Source: CAD feature listing. Evaluate the final solid. Frame: model axes, mm. Face numbers are marked on the shaded views. A direction names the side the tool comes from. Coordinates: 2 decimals unless noted, no trailing zeros. Order: outer loops, then holes, each group sorted by start corner. A loop starts at its lowest first (then second) coordinate and runs counter-clockwise, first axis right, second up.
Item 1: Mould query, pull axis X, two halves, no side actions, for the marked faces 4, 5 and 6. Classes: released by +X, released by -X, zero draft, split by the parting line, or undercut.
Item 2: Section B-B on z = 17. Return the cut outline in (x, y), then the cut area to 3 significant figures.
Item 3: Section A-A on y = 14.05. Return the cut outline in (x, z) (3 decimals), then the cut area to 3 significant figures.
Item 4: Ray query, line 1 (Z direction, x = 7.5, y = 13.6) (3 decimals); line 2 (Z direction, x = 5.5, y = 14.1); line 3 (Z direction, x = 6.75, y = 16.95). Return the intervals inside material, ascending.
Item 5: Section D-D on z = 13.25. Return the cut outline in (x, y).
Item 6: Section C-C on y = 15.3. Return the cut outline in (x, z) (3 decimals).
Item 7: Reachability of the marked faces 1, 2 and 3 from +Z, -Z, +X, -X, +Y, -Y: full face, straight path, thin tool, end or side. Return the list, or none.
Item 8: Contact query for flat-ended pins moving along their axis: P1, Ø8, axis at x = 12.5, z = -4.5, coming from the +Y side; P2, Ø4, axis at x = 8.6, z = 14.5, coming from the -Y side; P3, Ø0.9, axis at x = 12.5, y = 17, coming from the +Z side. Output: stop coordinate, or through.
from build123d import *

# Parameters (mm, degrees)
BOSS_EXTRUDE1_DEPTH  = 9
SKETCH6_W            = 16
SKETCH6_H            = 9
BOSS_EXTRUDE6_DEPTH  = 2.75
SKETCH7_W            = 16
SKETCH7_H            = 2.75
BOSS_EXTRUDE7_DEPTH  = 10
SKETCH8_W            = 16
SKETCH8_H            = 2.75
BOSS_EXTRUDE8_DEPTH  = 10
SKETCH10_R           = 1.625
CUT_EXTRUDE1_DEPTH   = 10
CUT_EXTRUDE2_DEPTH   = 1.5
BOSS_EXTRUDE11_DEPTH = 0.3


with BuildPart() as part:
    # Sketch1 → Boss-Extrude1 (new body)
    with BuildSketch(Plane.XY):
        with BuildLine():
            Line((16.338025278, 17.821295042), (16.597849853, 17.821295042))
            Line((16.597849853, 17.821295042), (16.597849853, 15.951295042))
            Line((16.597849853, 15.951295042), (0.597849853, 15.951295042))
            Line((0.597849853, 15.951295042), (0.597849853, 17.821295042))
            Line((0.597849853, 17.821295042), (0.857674428, 17.821295042))
            ThreePointArc((0.857674428, 17.821295042), (0.956581499, 17.784066453), (1.006392961, 17.690860259))
            ThreePointArc((1.006392961, 17.690860259), (1.040238138, 17.533232888), (1.098973448, 17.383092794))
            ThreePointArc((1.098973448, 17.383092794), (1.303700441, 17.155655983), (1.597849853, 17.071295042))
            ThreePointArc((1.597849853, 17.071295042), (1.891999264, 17.155655983), (2.096726257, 17.383092794))
            ThreePointArc((2.096726257, 17.383092794), (2.155461567, 17.533232888), (2.189306744, 17.690860259))
            ThreePointArc((2.189306744, 17.690860259), (2.239118207, 17.784066453), (2.338025278, 17.821295042))
            Line((2.338025278, 17.821295042), (2.857674428, 17.821295042))
            ThreePointArc((2.857674428, 17.821295042), (2.956581499, 17.784066453), (3.006392961, 17.690860259))
            ThreePointArc((3.006392961, 17.690860259), (3.040238138, 17.533232888), (3.098973448, 17.383092794))
            ThreePointArc((3.098973448, 17.383092794), (3.303700441, 17.155655983), (3.597849853, 17.071295042))
            ThreePointArc((3.597849853, 17.071295042), (3.891999264, 17.155655983), (4.096726257, 17.383092794))
            ThreePointArc((4.096726257, 17.383092794), (4.155461567, 17.533232888), (4.189306744, 17.690860259))
            ThreePointArc((4.189306744, 17.690860259), (4.239118207, 17.784066453), (4.338025278, 17.821295042))
            Line((4.338025278, 17.821295042), (4.857674428, 17.821295042))
            ThreePointArc((4.857674428, 17.821295042), (4.956581499, 17.784066453), (5.006392961, 17.690860259))
            ThreePointArc((5.006392961, 17.690860259), (5.040238138, 17.533232888), (5.098973448, 17.383092794))
            ThreePointArc((5.098973448, 17.383092794), (5.303700441, 17.155655983), (5.597849853, 17.071295042))
            ThreePointArc((5.597849853, 17.071295042), (5.891999264, 17.155655983), (6.096726257, 17.383092794))
            ThreePointArc((6.096726257, 17.383092794), (6.155461567, 17.533232888), (6.189306744, 17.690860259))
            ThreePointArc((6.189306744, 17.690860259), (6.239118207, 17.784066453), (6.338025278, 17.821295042))
            Line((6.338025278, 17.821295042), (6.857674428, 17.821295042))
            ThreePointArc((6.857674428, 17.821295042), (6.956581499, 17.784066453), (7.006392961, 17.690860259))
            ThreePointArc((7.006392961, 17.690860259), (7.040238138, 17.533232888), (7.098973448, 17.383092794))
            ThreePointArc((7.098973448, 17.383092794), (7.303700441, 17.155655983), (7.597849853, 17.071295042))
            ThreePointArc((7.597849853, 17.071295042), (7.891999264, 17.155655983), (8.096726257, 17.383092794))
            ThreePointArc((8.096726257, 17.383092794), (8.155461567, 17.533232888), (8.189306744, 17.690860259))
            ThreePointArc((8.189306744, 17.690860259), (8.239118207, 17.784066453), (8.338025278, 17.821295042))
            Line((8.338025278, 17.821295042), (8.857674428, 17.821295042))
            ThreePointArc((8.857674428, 17.821295042), (8.956581499, 17.784066453), (9.006392961, 17.690860259))
            ThreePointArc((9.006392961, 17.690860259), (9.040238138, 17.533232888), (9.098973448, 17.383092794))
            ThreePointArc((9.098973448, 17.383092794), (9.303700441, 17.155655983), (9.597849853, 17.071295042))
            ThreePointArc((9.597849853, 17.071295042), (9.891999264, 17.155655983), (10.096726257, 17.383092794))
            ThreePointArc((10.096726257, 17.383092794), (10.155461567, 17.533232888), (10.189306744, 17.690860259))
            ThreePointArc((10.189306744, 17.690860259), (10.239118207, 17.784066453), (10.338025278, 17.821295042))
            Line((10.338025278, 17.821295042), (10.857674428, 17.821295042))
            ThreePointArc((10.857674428, 17.821295042), (10.956581499, 17.784066453), (11.006392961, 17.690860259))
            ThreePointArc((11.006392961, 17.690860259), (11.040238138, 17.533232888), (11.098973448, 17.383092794))
            ThreePointArc((11.098973448, 17.383092794), (11.303700441, 17.155655983), (11.597849853, 17.071295042))
            ThreePointArc((11.597849853, 17.071295042), (11.891999264, 17.155655983), (12.096726257, 17.383092794))
            ThreePointArc((12.096726257, 17.383092794), (12.155461567, 17.533232888), (12.189306744, 17.690860259))
            ThreePointArc((12.189306744, 17.690860259), (12.239118207, 17.784066453), (12.338025278, 17.821295042))
            Line((12.338025278, 17.821295042), (12.857674428, 17.821295042))
            ThreePointArc((12.857674428, 17.821295042), (12.956581499, 17.784066453), (13.006392961, 17.690860259))
            ThreePointArc((13.006392961, 17.690860259), (13.040238138, 17.533232888), (13.098973448, 17.383092794))
            ThreePointArc((13.098973448, 17.383092794), (13.303700441, 17.155655983), (13.597849853, 17.071295042))
            ThreePointArc((13.597849853, 17.071295042), (13.891999264, 17.155655983), (14.096726257, 17.383092794))
            ThreePointArc((14.096726257, 17.383092794), (14.155461567, 17.533232888), (14.189306744, 17.690860259))
            ThreePointArc((14.189306744, 17.690860259), (14.239118207, 17.784066453), (14.338025278, 17.821295042))
            Line((14.338025278, 17.821295042), (14.857674428, 17.821295042))
            ThreePointArc((14.857674428, 17.821295042), (14.956581499, 17.784066453), (15.006392961, 17.690860259))
            ThreePointArc((15.006392961, 17.690860259), (15.040238138, 17.533232888), (15.098973448, 17.383092794))
            ThreePointArc((15.098973448, 17.383092794), (15.303700441, 17.155655983), (15.597849853, 17.071295042))
            ThreePointArc((15.597849853, 17.071295042), (15.891999264, 17.155655983), (16.096726257, 17.383092794))
            ThreePointArc((16.096726257, 17.383092794), (16.155461567, 17.533232888), (16.189306744, 17.690860259))
            ThreePointArc((16.189306744, 17.690860259), (16.239118207, 17.784066453), (16.338025278, 17.821295042))
        make_face()
    extrude(amount=BOSS_EXTRUDE1_DEPTH)

    # Sketch6 → Boss-Extrude6 (add)
    with BuildSketch(Plane.XZ.offset(-15.951295042)):
        with Locations((8.597849853, 4.5)):
            Rectangle(SKETCH6_W, SKETCH6_H)
    extrude(amount=BOSS_EXTRUDE6_DEPTH)

    # Sketch7 → Boss-Extrude7 (add)
    with BuildSketch(Plane(origin=(0, 0, 0), x_dir=(-1, 0, 0), z_dir=(0, 0, -1))):
        with Locations((-8.597849853, 14.576295042)):
            Rectangle(SKETCH7_W, SKETCH7_H)
    extrude(amount=BOSS_EXTRUDE7_DEPTH)

    # Sketch8 → Boss-Extrude8 (add)
    with BuildSketch(Plane.XY.offset(9)):
        with Locations((8.597849853, 14.576295042)):
            Rectangle(SKETCH8_W, SKETCH8_H)
    extrude(amount=BOSS_EXTRUDE8_DEPTH)

    # Sketch10 → Cut-Extrude1 (cut)
    with BuildSketch(Plane.XZ.offset(-13.201295042)):
        with Locations((8.597849853, 14.5)):
            Circle(SKETCH10_R)
        with Locations((8.597849853, -5.5)):
            Circle(SKETCH10_R)
    extrude(amount=-CUT_EXTRUDE1_DEPTH, mode=Mode.SUBTRACT)

    # Sketch11 → Cut-Extrude2 (cut)
    with BuildSketch(Plane.XZ.offset(-13.201295042)):
        Polygon((6.937967829, 11.625), (10.257731877, 11.625), (11.9176139, 14.5), (10.257731877, 17.375), (6.937967829, 17.375), (5.278085805, 14.5), align=None)
        Polygon((5.278085805, -5.5), (6.937967829, -2.625), (10.257731877, -2.625), (11.9176139, -5.5), (10.257731877, -8.375), (6.937967829, -8.375), align=None)
    extrude(amount=-CUT_EXTRUDE2_DEPTH, mode=Mode.SUBTRACT)

    # Sketch15 → Boss-Extrude11 (add)
    with BuildSketch(Plane.XZ.offset(-14.701295042)):
        Polygon((5.278085805, 14.5), (6.937967829, 11.625), (10.257731877, 11.625), (11.9176139, 14.5), (10.257731877, 17.375), (6.937967829, 17.375), align=None)
        Polygon((6.937967829, -8.375), (5.278085805, -5.5), (6.937967829, -2.625), (10.257731877, -2.625), (11.9176139, -5.5), (10.257731877, -8.375), align=None)
    extrude(amount=-BOSS_EXTRUDE11_DEPTH)


solid = part.part
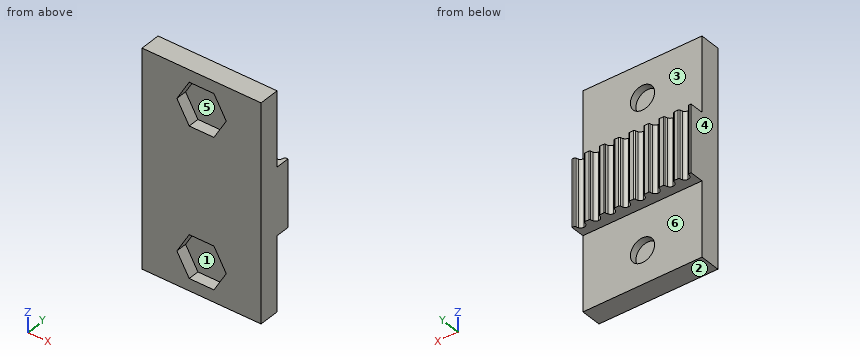
Answer list:
1. face 4: released by -X
1. face 5: undercut
1. face 6: zero draft
2. outline: (0.6, 13.2) - (6.72, 13.2) - (6.72, 14.7) - (10.47, 14.7) - (10.47, 13.2) - (16.6, 13.2) - (16.6, 15.95) - (0.6, 15.95) - close
2. area: 38.4 mm2
3. outline: (0.598, -10) - (16.598, -10) - (16.598, 19) - (0.598, 19) - close; hole (5.278, -5.5) - (6.938, -8.375) - (10.258, -8.375) - (11.918, -5.5) - (10.258, -2.625) - (6.938, -2.625) - close; hole (5.278, 14.5) - (6.938, 11.625) - (10.258, 11.625) - (11.918, 14.5) - (10.258, 17.375) - (6.938, 17.375) - close
3. area: 407 mm2
4. line 1: z = -10 to -8.375, -2.625 to 11.625, 17.375 to 19
4. line 2: z = -10 to -5.88, -5.12 to 14.12, 14.88 to 19
4. line 3: z = 0 to 9
5. outline: (0.6, 13.2) - (6, 13.2) - (6, 14.7) - (11.2, 14.7) - (11.2, 13.2) - (16.6, 13.2) - (16.6, 15.95) - (9.64, 15.95) - (9.64, 15) - (7.56, 15) - (7.56, 15.95) - (0.6, 15.95) - close
6. outline: (0.598, -10) - (16.598, -10) - (16.598, 19) - (0.598, 19) - close; hole circle Ø3.25 at (8.598, -5.5); hole circle Ø3.25 at (8.598, 14.5)
7. face 1: -Y
7. face 2: -Z, +X, -X, +Y, -Y
7. face 3: +Z, +X, -X, +Y
8. P1: stops at y = 15.95
8. P2: stops at y = 14.7
8. P3: stops at z = 9
